Can you work these out from the model? Positions are in its coordinate system, mm. A direction names the side the tool comes from. Round coordinates to 2 decimals unless told otherwise and drop trailing zeros. Write each loop counter-clockwise with the first axis right and the second up, starting at its lowest first coordinate (ties: lowest second). Pieces come first, ordered by that corner, then holes. Notation, with made-up numbers: (8.5, 60) - (23.5, 60) arc R27 cw to (23.5, 77) - close; hole circle Ø6 at (6, -28). An arc over 180 degrees is marked (long way). One line per item, written item: value. Start each with the question number.
(1) On a 3-axis mill with a long thin cutter (end or side, diameter ignored), from which of +Z, -Z, +X, -X, +Y, -Y can I reach the whole of each face in a straight line? I mean faces 5 (the face through (0.4, -4.8, 3.4)), 6 (the face through (-5, 3, 5)). Say none if no direction works.
(2) If I drill on L1, parallel to Y at x = 0, z = 2.5; L2, parallel to X at y = -6, z = 5; L3, parallel to Z at x = 0, y = -3.7, over which ranges is the centre line in solid material (lowest first)? Write a range as from..to.
(3) Thinking about a two-plate mould opening in Y: for faces 1 (the face through (-1.2, 3.1, 0)), 2 (the face through (0, 13, 5)), 3 (the face through (-0.397, 3.024, 4.93)), 4 (the face through (0, -7, 3)), which applies, +Y half, -Y half, draft (parallel to the pull), parting line (faces both ways), or undercut?
(4) I want a section at D-D on z = 1. List the corners of the cut face in (x, y) for me.
(5) I'm going to push a flat-ended pin straight in: pin 1 Ø2 at (x, y) = (0, 8) entering from -Z. Where does the tip first touch, or does it pass through?
(6) I want a section at A-A on z = 5. List the corners of the cut face in (x, y) for me.
(7) I want a section at C-C on y = 0. List the corners of the cut face in (x, z) for me.
(8) I want a section at B-B on x = 0. List the corners of the cut face in (y, z) for me.
from build123d import *

# Parameters (mm, degrees)
F0_W     = 10
F0_H     = 20
F0_R     = 3.05
F0_R_2   = 1.25
F1_DEPTH = 10
F3_D     = 3.3
F3_DEPTH = 7


with BuildPart() as f1:
    # F0 (on Top) → F1 (new body)
    with BuildSketch(Plane.XY):
        with Locations((0, 3)):
            Rectangle(F0_W, F0_H)
        Circle(F0_R, mode=Mode.SUBTRACT)
        with Locations((0, 8)):
            Circle(F0_R_2, mode=Mode.SUBTRACT)
    extrude(amount=F1_DEPTH)

    # F3
    with Locations(Plane.XZ.offset(7)):
        with Locations((0, 5)):
            Hole(F3_D / 2, depth=F3_DEPTH)


solid = f1.part
Established:
1. face 5: -Y
1. face 6: +Z, -Z, -X, +Y, -Y
2. L1: -7..-3.05, 3.05..6.75, 9.25..13
2. L2: -5..-1.65, 1.65..5
2. L3: 0..3.35, 6.65..10
3. face 1: draft
3. face 2: +Y half
3. face 3: undercut
3. face 4: -Y half
4. outline: (-5, -7) - (5, -7) - (5, 13) - (-5, 13) - close; hole circle Ø6.1 at (0, 0); hole circle Ø2.5 at (0, 8)
5. pin 1: through
6. outline: (-5, -7) - (-1.65, -7) - (-1.65, -2.57) arc R3.05 cw (long way) to (1.65, -2.57) - (1.65, -7) - (5, -7) - (5, 13) - (-5, 13) - close; hole circle Ø2.5 at (0, 8)
7. outline: (-5, 0) - (-3.05, 0) - (-3.05, 10) - (-5, 10) - close; (3.05, 0) - (5, 0) - (5, 10) - (3.05, 10) - close
8. outline: (-7, 0) - (-3.05, 0) - (-3.05, 3.35) - (-7, 3.35) - close; (-7, 6.65) - (-3.05, 6.65) - (-3.05, 10) - (-7, 10) - close; (3.05, 0) - (6.75, 0) - (6.75, 10) - (3.05, 10) - close; (9.25, 0) - (13, 0) - (13, 10) - (9.25, 10) - close
